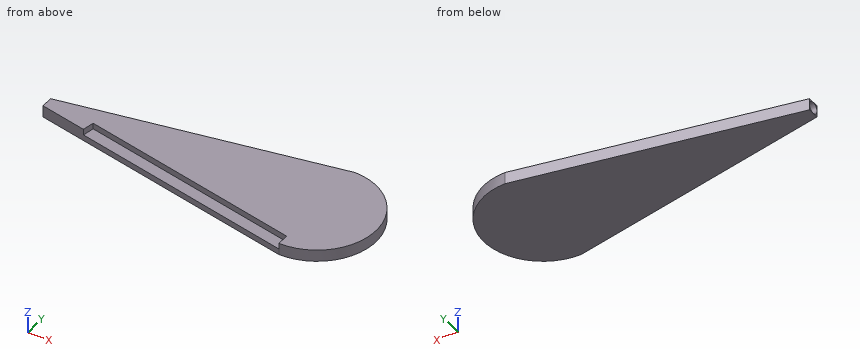
```python
from build123d import *

# Parameters (mm, degrees)
F0_W     = 177.8
F0_H     = 63.5
F1_DEPTH = 6.35
F3_DEPTH = 25.4
F5_DEPTH = 25.4
F6_R     = 3.1115
F7_DEPTH = 25.4
F9_DEPTH = 3.175


# Not quite as in the source:
# - ends of sketch curves that miss each other by under 0.0002 mm in the source are joined


with BuildPart() as f1:
    # F0 (on Top) → F1 (new body)
    with BuildSketch(Plane.XY):
        with Locations((88.9, 31.75)):
            Rectangle(F0_W, F0_H)
    extrude(amount=F1_DEPTH)

    # F2 (on face) → F3 (cut)
    with BuildSketch(Plane.XY.offset(6.35)):
        with BuildLine():
            ThreePointArc((146.05, 63.5), (168.5006403027, 54.2006403027), (177.8, 31.75))
            Line((177.8, 31.75), (177.8, 63.5))
            Line((177.8, 63.5), (146.05, 63.5))
        make_face()
        with BuildLine():
            ThreePointArc((177.8, 31.75), (168.5006402649, 9.2993596596), (146.0499998933, 0))
            Line((146.0499998933, 0), (177.8, 0))
            Line((177.8, 0), (177.8, 31.75))
        make_face()
    extrude(amount=-F3_DEPTH, mode=Mode.SUBTRACT)

    # F4 (on face) → F5 (cut)
    with BuildSketch(Plane.XY.offset(6.35)):
        Polygon((0, 34.925), (146.05, 63.5), (0, 63.5), align=None)
        Polygon((0, 0), (146.0499998933, 0), (0, 28.575), align=None)
    extrude(amount=-F5_DEPTH, mode=Mode.SUBTRACT)

    # F6 (on face) → F7 (cut)
    with BuildSketch(Plane(origin=(0, 0, 0), x_dir=(0, -1, 0), z_dir=(-1, 0, 0))):
        with Locations((-31.75, 3.175)):
            Circle(F6_R)
    extrude(amount=-F7_DEPTH, mode=Mode.SUBTRACT)

    # F8 (on face) → F9 (cut)
    with BuildSketch(Plane.XY.offset(6.35)):
        Polygon((26.2400177438, 29.9114803934), (25.0207440433, 23.679637035), (146.05, 0), (146.05, 6.4703969085), align=None)
    extrude(amount=-F9_DEPTH, mode=Mode.SUBTRACT)


solid = f1.part
```
Could you check a few things on this model? Use its own coordinates, in mm. Round coordinates to 2 decimals unless told otherwise and drop trailing zeros. Loops run counter-clockwise (first coordinate to the right, second up) from the corner with the lowest first, then second, coordinate; pieces in that order, holes last. Notation, with made-up numbers: M -20,-39 L -8,-39 A21 cw -8,-9 Z; hole C 44.5,10 d10. An arc over 180 degrees is marked long. Write item = value, one per line.
1. Will these pins go through, and if not, where does the flat tip stop? P1, Ø1.5, axis at x = 66, z = 4, coming from the -Y side; P2, Ø8, axis at x = 92, y = 12.5, coming from the +Z side (3 decimals); P3, Ø2.5, axis at y = 3.5, z = 5, coming from the -X side.
Results below:
P1 = 21.99
P2 = 3.175
P3 = 146.05
2. I want a section at D-D, the plane x = 45. Write out the boundary of the cut face in (y, z) (3 decimals), and give its area (3 significant figures).
Results below:
outline = M 19.771,0 L 43.729,0 L 43.729,6.35 L 26.241,6.35 L 26.241,3.175 L 19.771,3.175 Z
area = 132 mm²
3. I want a section at A-A, the plane y = 31.75. Write out the boundary of the cut face in (x, z), and give its area (3 significant figures).
Results below:
outline = M 0,0 L 177.8,0 L 177.8,6.35 L 0,6.35 L 0,6.29 L 25.4,6.29 L 25.4,0.06 L 0,0.06 Z
area = 971 mm²
4. I want a section at B-B, the plane z = 4.5. Write out the boundary of the cut face in (x, y) (3 decimals).
Results below:
outline = M 0,28.575 L 25.021,23.68 L 26.24,29.911 L 146.05,6.47 L 146.05,0 A31.75 ccw 146.05,63.5 L 0,34.925 L 0,34.565 L 25.4,34.565 L 25.4,28.935 L 0,28.935 Z
5. I need wall thicknesses on probe 1 along X at (y, z) = (32.5, 1.5); probe 2 along Y at (x, z) = (68, 3.5); probe 3 along Y at (x, z) = (114.5, 6.25). Which ranges of each line are inside material? Lowest first, please.
Results below:
probe_1 = 25.4 to 177.79
probe_2 = 21.74 to 48.23
probe_3 = 12.64 to 57.33
